The listing builds one solid part. Answer for the finished solid, in the listing's coordinates (mm). A direction names the side the tool comes from. Coordinates: 2 decimals unless noted, no trailing zeros. Order: outer loops, then holes, each group sorted by start corner. A loop starts at its lowest first (then second) coordinate and runs counter-clockwise, first axis right, second up.
from build123d import *

# Parameters (mm, degrees)
BOSS_EXTRUDE1_DEPTH = 1
SKETCH3_R           = 2
BOSS_EXTRUDE2_DEPTH = 1
BOSS_EXTRUDE3_DEPTH = 3
SKETCH5_R           = 1.5
BOSS_EXTRUDE6_DEPTH = 8


with BuildPart() as part:
    # Sketch2 → Boss-Extrude1 (new body)
    with BuildSketch(Plane.XY):
        Polygon((-12, -2), (-12, 2), (-8, 8), (0, 8), (0, -8), (-8, -8), align=None)
    boss_extrude1 = extrude(amount=BOSS_EXTRUDE1_DEPTH)

    # Sketch3 → Boss-Extrude2 (add)
    with BuildSketch(Plane.XY.offset(1)):
        with Locations((-4, -4)):
            Circle(SKETCH3_R)
        with Locations(Location((-4, 4, 0), (0, 0, 180))):
            Circle(SKETCH3_R)
    boss_extrude2 = extrude(amount=BOSS_EXTRUDE2_DEPTH)

    # Sketch4 → Boss-Extrude3 (add)
    with BuildSketch(Plane.XY.offset(1)):
        Polygon((-12, -2), (-8, -8), (-8, -6.197224362), (-11, -1.697224362), (-11, 1.697224362), (-8, 6.197224362), (-8, 8), (-12, 2), align=None)
    boss_extrude3 = extrude(amount=BOSS_EXTRUDE3_DEPTH)

    # Sketch5 → Boss-Extrude6 (add)
    with BuildSketch(Plane.ZY.offset(12)):
        with Locations(Location((2, 0, 0), (0, 0, 180))):
            Circle(SKETCH5_R)
    boss_extrude6 = extrude(amount=BOSS_EXTRUDE6_DEPTH)

    # Mirror3: Boss-Extrude1, Boss-Extrude2, Boss-Extrude3, Boss-Extrude6 across plane
    add(boss_extrude1.mirror(Plane(origin=(0, 0, 0), x_dir=(0, 0, 1), z_dir=(1, 0, 0))))
    add(boss_extrude2.mirror(Plane(origin=(0, 0, 0), x_dir=(0, 0, 1), z_dir=(1, 0, 0))))
    add(boss_extrude3.mirror(Plane(origin=(0, 0, 0), x_dir=(0, 0, 1), z_dir=(1, 0, 0))))
    add(boss_extrude6.mirror(Plane(origin=(0, 0, 0), x_dir=(0, 0, 1), z_dir=(1, 0, 0))))


solid = part.part
1) Section B-B (x = -4) is taken. Give the vertices of the cut face in (y, z).
2) Section A-A (z = 2.95) is taken. Give the vertices of the cut face in (x, y), then the cut area to 3 significant figures.
3) Consider L1, parallel to X at y = 0.5, z = 3.6; L2, parallel to X at y = -0.25, z = 2.95; L3, parallel to Z at x = 3, y = 5.5. Determine where each line is inside the solid, lowest interval first.
4) Section C-C (y = 0) is taken. Give the vertices of the cut face in (x, z), then the cut area to 3 significant figures.
5) Section D-D (x = -8.5) is taken. Give the vertices of the cut face in (y, z).
6) Each of these flat-tipped pins is pushed along its axis until it touches: P1, Ø4.5, axis at x = 4.5, y = -4, coming from the +Z side; P2, Ø1.4, axis at y = -7, z = 3, coming from the -X side; P3, Ø1.4, axis at y = 7.5, z = 2.5, coming from the -X side. Where does it stop, or does it pass through?
7) A tool of negligible diameter and unlimited length cuts with its end or side. For faces 1 (the face through (-11, 0, 2)), 2 (the face through (15.94, -0.45, 0.57)), 3 (the face through (-0.1, -8, 0.5)), 4 (the face through (-4, -4, 2)), from which of +Z, -Z, +X, -X, +Y, -Y can it reach the whole face along a straight path? Write none if from no direction.
8) Determine the mould class of faces 5 (the face through (0, 0, 1)), 6 (the face through (-20, 0, 2)), 7 (the face through (-15.94, -0.45, 0.57)), 8 (the face through (2.4, 5.2, 1.5)) for opening direction X: released by +X, released by -X, zero draft, split by the parting line, or undercut.
Filled sheet:
1. outline: (-8, 0) - (8, 0) - (8, 1) - (6, 1) - (6, 2) - (2, 2) - (2, 1) - (-2, 1) - (-2, 2) - (-6, 2) - (-6, 1) - (-8, 1) - close
2. outline: (-20, -1.16) - (-12, -1.16) - (-12, -2) - (-8, -8) - (-8, -6.2) - (-11, -1.7) - (-11, 1.7) - (-8, 6.2) - (-8, 8) - (-12, 2) - (-12, 1.16) - (-20, 1.16) - close; (8, -8) - (12, -2) - (12, -1.16) - (20, -1.16) - (20, 1.16) - (12, 1.16) - (12, 2) - (8, 8) - (8, 6.2) - (11, 1.7) - (11, -1.7) - (8, -6.2) - close
2. area: 69.8 mm2
3. L1: x = -12 to -11, 11 to 12
3. L2: x = -20 to -11, 11 to 20
3. L3: z = 0 to 2
4. outline: (-20, 0.5) - (-12, 0.5) - (-12, 0) - (12, 0) - (12, 0.5) - (20, 0.5) - (20, 3.5) - (12, 3.5) - (12, 4) - (11, 4) - (11, 1) - (-11, 1) - (-11, 4) - (-12, 4) - (-12, 3.5) - (-20, 3.5) - close
4. area: 78.0 mm2
5. outline: (-7.25, 0) - (7.25, 0) - (7.25, 4) - (5.45, 4) - (5.45, 1) - (-5.45, 1) - (-5.45, 4) - (-7.25, 4) - close
6. P1: stops at z = 2
6. P2: stops at x = -9.13
6. P3: stops at x = -8.8
7. face 1: +Z
7. face 2: +X
7. face 3: +Z, -Z, +X, -X, -Y
7. face 4: +Z, +Y, -Y
8. face 5: undercut
8. face 6: released by -X
8. face 7: zero draft
8. face 8: undercut
